from build123d import *

# Parameters (mm, degrees)
BOSS_EXTRUDE3_DEPTH   = 4
BOSS_EXTRUDE4_DEPTH   = 15.45
M3X0_5_TAPPED_HOLE1_D = 2.5


with BuildPart() as part:
    # Sketch1 → Boss-Extrude3 (new, symmetric)
    with BuildSketch(Plane.XY):
        with BuildLine():
            Line((0, 0), (0, 15.45))
            Line((0, 15.45), (-5.55, 15.45))
            Line((-5.55, 15.45), (-5.55, 8.5))
            ThreePointArc((-5.55, 8.5), (-5.696446609, 8.146446609), (-6.05, 8))
            Line((-6.05, 8), (-21.05, 8))
            Line((-21.05, 8), (-21.05, 3))
            Line((-21.05, 3), (-6.05, 3))
            ThreePointArc((-6.05, 3), (-5.696446609, 2.853553391), (-5.55, 2.5))
            Line((-5.55, 2.5), (-5.55, 0))
            Line((-5.55, 0), (0, 0))
        make_face()
    extrude(amount=BOSS_EXTRUDE3_DEPTH, both=True)

    # Sketch2 → Boss-Extrude4 (add)
    with BuildSketch(Plane.XZ):
        with BuildLine():
            Line((-0.875, 4), (-2.875, 4))
            ThreePointArc((-2.875, 4), (-1.875, 5), (-0.875, 4))
        make_face()
        with BuildLine():
            Line((-0.875, -4), (-2.875, -4))
            ThreePointArc((-2.875, -4), (-1.875, -5), (-0.875, -4))
        make_face()
    extrude(amount=-BOSS_EXTRUDE4_DEPTH)

    # M3x0.5 Tapped Hole1 (through all)
    with Locations(Plane(origin=(0, 3, 0), x_dir=(-1, 0, 0), z_dir=(0, -1, 0))):
        with Locations((17.05, 0), (10.05, 0)):
            Hole(M3X0_5_TAPPED_HOLE1_D / 2)


solid = part.part
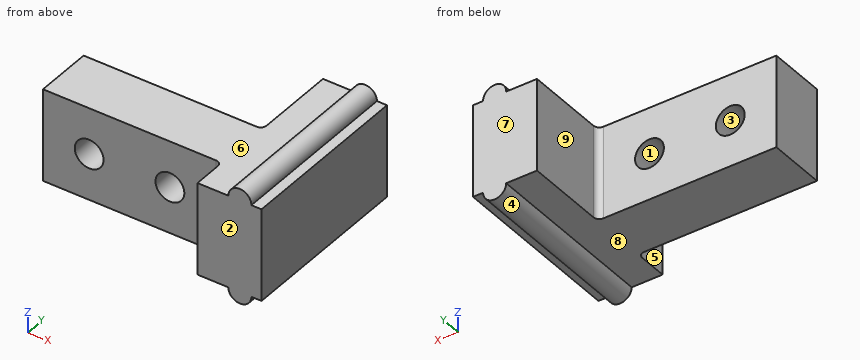
The model under review builds one solid part; all positions refer to its coordinate system, in mm. Face numbers are marked on the shaded views. A direction names the side the tool comes from. Round coordinates to 2 decimals unless told otherwise and drop trailing zeros. Order: outer loops, then holes, each group sorted by start corner. A loop starts at its lowest first (then second) coordinate and runs counter-clockwise, first axis right, second up. Notation, with made-up numbers: (50, 20.5) -> (74, 20.5) arc R20 ccw to (74, 40.5) -> close; hole circle Ø11 at (-18, -22). An arc over 180 degrees is marked (long way). Write item = value, one per line. Start each with the question number.
Item 1: Consider section B-B on y = 5.25. Write out the cut boundary in (x, z) (3 decimals).
Item 2: Consider section D-D on y = 1.5. Write out the cut boundary in (x, z) (3 decimals).
Item 3: Mouldability with a two-part tool opening along Z and no side actions: class the marked faces 1, 2, 3 and 4 as released by +Z, released by -Z, zero draft, split by the parting line, or undercut.
Item 4: Consider section A-A on x = -10.05. Write out the cut boundary in (y, z).
Item 5: Consider section C-C on z = 0. Write out the cut boundary in (x, y).
Item 6: Clearance check with flat-ended pins moving along their axes: pin 1 Ø5 at (x, y) = (-14, 7) entering from -Z; pin 2 Ø3 at (x, z) = (-10.05, 0) entering from +Y; pin 3 Ø5.5 at (y, z) = (12.5, -1.5) entering from -X. State where each tip first meets the part, or that it passes through.
Item 7: For line 1 along Z through (x, y) = (-17.05, 5.2); line 2 along X through (y, z) = (6, -1); line 3 along X through (y, z) = (3.25, 0.25), list the stretches that pass through material, from the lowest coordinate up.
Item 8: For the marked faces 5, 6, 7, 8 and 9, list the 3-axis set-ups (+Z, -Z, +X, -X, +Y, -Y) from which the entire face can be reached by the end or side of a thin tool; tool diameter is ignored.
Conclusion:
q1.outline = (-21.05, -4) -> (-2.875, -4) arc R1 ccw to (-0.875, -4) -> (0, -4) -> (0, 4) -> (-0.875, 4) arc R1 ccw to (-2.875, 4) -> (-21.05, 4) -> close; hole circle Ø2.5 at (-17.05, 0); hole circle Ø2.5 at (-10.05, 0)
q2.outline = (-5.55, -4) -> (-2.875, -4) arc R1 ccw to (-0.875, -4) -> (0, -4) -> (0, 4) -> (-0.875, 4) arc R1 ccw to (-2.875, 4) -> (-5.55, 4) -> close
q3.face_1 = undercut
q3.face_2 = zero draft
q3.face_3 = undercut
q3.face_4 = released by -Z
q4.outline = (3, -4) -> (8, -4) -> (8, -1.25) -> (3, -1.25) -> close; (3, 1.25) -> (8, 1.25) -> (8, 4) -> (3, 4) -> close
q5.outline = (-21.05, 3) -> (-18.3, 3) -> (-18.3, 8) -> (-21.05, 8) -> close; (-15.8, 3) -> (-11.3, 3) -> (-11.3, 8) -> (-15.8, 8) -> close; (-8.8, 3) -> (-6.05, 3) arc R0.5 cw to (-5.55, 2.5) -> (-5.55, 0) -> (0, 0) -> (0, 15.45) -> (-5.55, 15.45) -> (-5.55, 8.5) arc R0.5 cw to (-6.05, 8) -> (-8.8, 8) -> close
q6.pin_1 = -4
q6.pin_2 = 8
q6.pin_3 = -5.55
q7.line_1 = -4 to -1.25, 1.25 to 4
q7.line_2 = -21.05 to -17.8, -16.3 to -10.8, -9.3 to 0
q7.line_3 = -21.05 to -18.27, -15.83 to -11.27, -8.83 to 0
q8.face_5 = +Z, -Z, -X, -Y
q8.face_6 = +Z, -X, +Y, -Y
q8.face_7 = +Z, -Z, +X, -X, +Y
q8.face_8 = -Z, -X, +Y, -Y
q8.face_9 = +Z, -Z, -X, +Y
